Source: CAD feature listing. Evaluate the final solid. Frame: model axes, mm. A direction names the side the tool comes from. Coordinates: 2 decimals unless noted, no trailing zeros. Order: outer loops, then holes, each group sorted by start corner. A loop starts at its lowest first (then second) coordinate and runs counter-clockwise, first axis right, second up.
Autodesk Inventor part; units mm, degrees
ref_plane "YZ Plane" through (0, 0, 0) normal (1, 0, 0) x (0, 1, 0)
ref_plane "XZ Plane" through (0, 0, 0) normal (0, 1, 0) x (-1, 0, 0)
ref_plane "XY Plane" through (0, 0, 0) normal (0, 0, 1) x (1, 0, 0)
sketch "Sketch1" plane through (0, 0, 0) normal (0, 1, 0) x (-1, 0, 0)
  line L0 (19.05, -83) -> (19.05, 83)
  line L1 (-19.05, 83) -> (-19.05, -83)
  circle A0 centre (0, 0) radius 11.5094
  line L2 (0, 0) -> (-0.4877, 3.251) construction
  line L3 (0, 0) -> (0, 44.45) construction
  line L4 (0, 0) -> (0, -44.45) construction
  circle A1 centre (0, 44.45) radius 3.5719
  circle A2 centre (0, -44.45) radius 3.5719
  line L5 (19.05, 83) -> (-19.05, 83)
  line L6 (19.05, -83) -> (-19.05, -83)
  dimension "d2" = 23.0188
  dimension "d4" = 44.45
  dimension "d5" = 44.45
  dimension "d6" = 7.1437
  dimension "d7" = 7.1437
extrude "Extrusion1" add sketch "Sketch1" along normal blind 25.4
sketch "Sketch6" plane through (0, 0, 0) normal (0, -1, 0) x (1, 0, 0)
  circle A0 centre (0, 44.45) radius 3.5719
  circle A1 centre (0, 44.45) radius 3.5719
  circle A2 centre (0, -44.45) radius 3.5719
  circle A3 centre (0, -44.45) radius 3.5719
  circle A4 centre (0, 0) radius 5.1594
  circle A5 centre (0, 0) radius 11.5094
  dimension "d102" = 35.7188
sketch "Sketch13" plane through (0, 25.4, 0) normal (0, 1, 0) x (1, 0, 0)
  line L0 (-19.05, -83) -> (19.05, -83) construction
  line L1 (19.05, 83) -> (-19.05, 83) construction
  circle A0 centre (8.0969, -34) radius 1.8
  circle A1 centre (8.0969, -27) radius 1.8
  circle A2 centre (8.0969, -20) radius 1.8
  circle A3 centre (8.0969, 20) radius 1.8
  circle A4 centre (8.0969, 27) radius 1.8
  circle A5 centre (8.0969, 34) radius 1.8
  circle A6 centre (0, 0) radius 11.5094
  line L2 (-19.05, 83) -> (-19.05, -83)
  line L3 (-19.05, -83) -> (-13.0969, -83)
  line L4 (-13.0969, -83) -> (-13.0969, 83)
  line L5 (-13.0969, 83) -> (-19.05, 83)
  line L6 (-19.05, 83) -> (-19.05, -83)
  line L7 (19.05, -83) -> (13.0969, -83)
  line L8 (13.0969, -83) -> (13.0969, 83)
  line L9 (13.0969, 83) -> (19.05, 83)
  line L10 (19.05, 83) -> (19.05, -83)
  line L11 (13.0969, -83) -> (3.0969, -83) construction
  line L12 (3.0969, -83) -> (3.0969, 83) construction
  line L13 (3.0969, 83) -> (13.0969, 83) construction
  line L14 (13.0969, 83) -> (13.0969, -83) construction
  line L15 (8.0969, -83) -> (8.0969, 83) construction
  dimension "d82" = 3.6
  dimension "d83" = 3.6
  dimension "d84" = 3.6
  dimension "d85" = 3.6
  dimension "d86" = 3.6
  dimension "d87" = 3.6
  dimension "d88" = 7
  dimension "d89" = 7
  dimension "d90" = 7
  dimension "d92" = 7
  dimension "d93" = 20
  dimension "d94" = 20
  dimension "d97" = 1.5875
  dimension "d99" = 1.5875
  dimension "d105" = 10
sketch "Sketch14" plane through (19.05, 0, -83) normal (0, 0, -1) x (-1, 0, 0)
  line L0 (0, 0) -> (0, 25.4)
  line L1 (38.1, 0) -> (38.1, 25.4)
  line L2 (0, 25.4) -> (38.1, 25.4)
  line L3 (38.1, 25.4) -> (38.1, 16.2292)
  line L4 (38.1, 16.2292) -> (0, 16.2292)
  line L5 (0, 16.2292) -> (0, 25.4)
  point P0 (19.05, 0)
extrude "Extrusion15" cut sketch "Sketch14" against normal up to next
sketch "Sketch15" plane through (-19.05, 16.2292, -83) normal (0, 1, 0) x (1, 0, 0)
  line L0 (38.1, -166) -> (0, -166)
  line L1 (38.1, 0) -> (38.1, -166)
  line L2 (0, -166) -> (38.1, -166)
  line L3 (38.1, -166) -> (38.1, -134.1969)
  line L4 (38.1, -134.1969) -> (0, -134.1969)
  line L5 (0, -134.1969) -> (0, -166)
  circle A0 centre (19.05, -127.45) radius 3.5719
  line L6 (0, -166) -> (0, 0)
  line L7 (0, 0) -> (38.1, 0)
  line L8 (38.1, 0) -> (38.1, -31.8031)
  line L9 (38.1, -31.8031) -> (0, -31.8031)
  line L10 (0, -31.8031) -> (0, 0)
  circle A1 centre (19.05, -38.55) radius 3.5719
  point P0 (19.05, -83)
  dimension "d78" = 3.175
  dimension "d79" = 3.175
extrude "Extrusion16" cut sketch "Sketch15" against normal up to next contours L0 L5 L4 L1 | L9 L6 L7 L1
extrude "Extrusion18" cut sketch "Sketch13" against normal up to next contours A0 | A1 | A2 | A3 | A4 | A5 | L5 L4 L3 L2 | L7 L8 L9 L10
extrude "Extrusion19" add sketch "Sketch6" against normal blind 5 contours A0 | A2 | A4 | A5
properties part number "RodBase"
Q1. Pull-direction query (Z, two-part tool) for faces 1 (the cylindrical face through (0.465, 10.536, 40.908)), 2 (the flat face through (0, 8, -51.197)), 3 (the flat face through (0, 16.229, -12)); classes: pulls with the +Z half, pulls with the -Z half, needs draft (parallel to the pull), parting line crosses it, or undercut.
Solutions:
face 1: undercut
face 2: pulls with the -Z half
face 3: needs draft
Q2. Material intervals for line 1 along Z through (x, y) = (0, 10.75); line 2 along X through (y, z) = (9, -27); line 3 along Y through (x, z) = (-1, -45), sorted ascending.
Solutions:
line 1: z = -51.2 to -48.02, -40.88 to -11.51, 11.51 to 40.88, 48.02 to 51.2
line 2: x = -13.1 to 6.3, 9.9 to 13.1
line 3: y = 0 to 5
Q3. Section query B-B on y = 1.25. Output: boundary loops of the cut face in (x, z), plus the area to 3 significant figures.
Solutions:
outline: (-13.1, -51.2) - (13.1, -51.2) - (13.1, 51.2) - (-13.1, 51.2) - close; hole circle Ø3.6 at (8.1, -34); hole circle Ø3.6 at (8.1, -27); hole circle Ø3.6 at (8.1, -20); hole circle Ø3.6 at (8.1, 20); hole circle Ø3.6 at (8.1, 27); hole circle Ø3.6 at (8.1, 34)
area: 2,620 mm2
Q4. Set-up query: faces 4 (the cylindrical face through (-1.65, 10.54, -41.28)), 5 (the cylindrical face through (6.77, 8.228, 18.783)). Return all of +Z, -Z, +X, -X, +Y, -Y with unobstructed straight access to the full face (end or side cutting, diameter ignored); none if empty.
Solutions:
face 4: +Y
face 5: +Y, -Y
Q5. Section query A-A on y = 10.25. Give the number of separate pieces and of enclosed holes in the cut face, plus the area to 3 significant figures.
Solutions:
separate pieces: 1
enclosed holes: 9
area: 2,120 mm2
Q6. Section query C-C on z = 27. Output: boundary loops of the cut face in (x, y).
Solutions:
outline: (-13.1, 0) - (6.3, 0) - (6.3, 16.23) - (-13.1, 16.23) - close; (9.9, 0) - (13.1, 0) - (13.1, 16.23) - (9.9, 16.23) - close
Q7. Pin query (flat end, axial travel): P1, Ø2, axis at x = 8.1, z = -27, coming from the +Y side; P2, Ø3.5, axis at x = -1.5, z = 43.5, coming from the +Y side. Return the tip coordinate at first contact, or that it passes through.
Solutions:
P1: passes through
P2: stops at y = 5
